Geometry check sheet. Reference: the model listing, model coordinates, mm. A direction names the side the tool comes from. Give positions to 0.01 mm unless a question says otherwise; leave off trailing zeros. Write each loop counter-clockwise with the first axis right and the second up, starting at its lowest first coordinate (ties: lowest second). Pieces come first, ordered by that corner, then holes. Notation, with made-up numbers: (-38, 32.5) -> (-19, 32.5) arc R15 ccw to (-19, 55.5) -> close; hole circle Ø6 at (-32.5, 78). An arc over 180 degrees is marked (long way). Use a Markdown table: item, result. Add a question column.
from build123d import *

# Parameters (mm, degrees)
SKETCH1_W           = 94
SKETCH1_H           = 130
BOSS_EXTRUDE1_DEPTH = 30
CUT_EXTRUDE2_DEPTH  = 23
SKETCH7_W           = 72
SKETCH7_H           = 24
CUT_EXTRUDE3_DEPTH  = 164.205392068
SKETCH8_W           = 6
SKETCH8_H           = 18
CUT_EXTRUDE4_DEPTH  = 4
SKETCH9_W           = 43
SKETCH9_H           = 8
CUT_EXTRUDE5_DEPTH  = 2.5
SKETCH10_W          = 70
SKETCH10_H          = 78
CUT_EXTRUDE6_DEPTH  = 2
SKETCH11_W          = 23
SKETCH11_H          = 3.5
CUT_EXTRUDE7_DEPTH  = 163.849623887
FILLET1_R           = 2
SKETCH12_R          = 5
CUT_EXTRUDE8_DEPTH  = 10


with BuildPart() as part:
    # Sketch1 → Boss-Extrude1 (new body)
    with BuildSketch(Plane(origin=(0, 0, 0), x_dir=(1, 0, 0), z_dir=(0, 1, 0))):
        with Locations((47, 65)):
            Rectangle(SKETCH1_W, SKETCH1_H)
    extrude(amount=BOSS_EXTRUDE1_DEPTH)

    # Sketch6 → Cut-Extrude2 (cut)
    with BuildSketch(Plane.XZ):
        Polygon((84, -125), (84, -120), (89, -120), (89, -10), (84, -10), (84, -5), (10, -5), (10, -10), (5, -10), (5, -120), (10, -120), (10, -125), align=None)
    extrude(amount=-CUT_EXTRUDE2_DEPTH, mode=Mode.SUBTRACT)

    # Sketch7 → Cut-Extrude3 (cut, through all)
    with BuildSketch(Plane(origin=(0, 30, 0), x_dir=(1, 0, 0), z_dir=(0, 1, 0))):
        with Locations((47, 100)):
            Rectangle(SKETCH7_W, SKETCH7_H)
    extrude(amount=-CUT_EXTRUDE3_DEPTH, mode=Mode.SUBTRACT)

    # Sketch8 → Cut-Extrude4 (cut)
    with BuildSketch(Plane.XZ.offset(-23)):
        with Locations((86, -100)):
            Rectangle(SKETCH8_W, SKETCH8_H)
    extrude(amount=-CUT_EXTRUDE4_DEPTH, mode=Mode.SUBTRACT)

    # Sketch9 → Cut-Extrude5 (cut)
    with BuildSketch(Plane.XZ.offset(-23)):
        with Locations((33.5, -116)):
            Rectangle(SKETCH9_W, SKETCH9_H)
    extrude(amount=-CUT_EXTRUDE5_DEPTH, mode=Mode.SUBTRACT)

    # Sketch10 → Cut-Extrude6 (cut)
    with BuildSketch(Plane(origin=(0, 30, 0), x_dir=(1, 0, 0), z_dir=(0, 1, 0))):
        with Locations((42, 44)):
            Rectangle(SKETCH10_W, SKETCH10_H)
    extrude(amount=-CUT_EXTRUDE6_DEPTH, mode=Mode.SUBTRACT)

    # Sketch11 → Cut-Extrude7 (cut, through all)
    with BuildSketch(Plane(origin=(0, 28, 0), x_dir=(1, 0, 0), z_dir=(0, 1, 0))):
        with Locations((42, 9.25)):
            Rectangle(SKETCH11_W, SKETCH11_H)
    extrude(amount=-CUT_EXTRUDE7_DEPTH, mode=Mode.SUBTRACT)

    # Fillet1
    fillet1_edges = [part.edges().sort_by_distance(p)[0] for p in [
        (94, 30, -65),
        (47, 30, -130),
        (0, 30, -65),
        (47, 30, 0),
        (0, 15, -130),
        (94, 15, -130),
        (94, 15, 0),
        (0, 15, 0),
    ]]
    fillet(fillet1_edges, radius=FILLET1_R)

    # Sketch12 → Cut-Extrude8 (cut)
    with BuildSketch(Plane.XY):
        with Locations((17.400096769, 12)):
            Circle(SKETCH12_R)
    extrude(amount=-CUT_EXTRUDE8_DEPTH, mode=Mode.SUBTRACT)


solid = part.part
1) Draft check along Z on faces 1 (the face through (30.5, 26, -9)), 2 (the face through (89, 13, -66)), 3 (the face through (46, 14, 0)), 4 (the face through (2, 0, -65)). Enter one of: +Z half, -Z half, draft (parallel to the pull), parting line (faces both ways), or undercut.
2) Sectioned sample at D-D, the plane z = -70. Enter the section's corners in (x, y), and give its area (3 significant figures).
3) Tool access check on faces 5 (the face through (33, 24, -120)), 6 (the face through (0, 14, -64)), 7 (the face through (42, 28, -45)), 8 (the face through (42, 26, -7.5)), 9 (the face through (47, 30, -84)). Record the directions out of +Z, -Z, +X, -X, +Y, -Y that give a thin tool (end or side, any length) a straight path to the whole face; none if there is none.
4) Sectioned sample at A-A, the plane x = 73. Enter the section's corners in (y, z).
5) Sectioned sample at B-B, the plane x = 32. Enter the section's corners in (y, z), and give its area (3 significant figures).
6) Material ranges on probe 1 along Z at (x, y) = (27, 16); probe 2 along X at (y, z) = (1.75, -34.5); probe 3 along X at (y, z) = (19.75, -7.5), recorded low to high. Write a range as [from, to].
7) Gauge pin test, flat ends, axial feed: P1, Ø0.6, axis at y = 29, z = -54.5, coming from the -X side; P2, Ø0.8, axis at x = 34.5, y = 24, coming from the +Z side. Record the tip position at first contact, or that the pin passes through.
8) Sectioned sample at C-C, the plane y = 3. Enter the section's corners in (x, z).
Check values:
| question | item | result |
|---|---|---|
| 1 | face 1 | undercut |
| 1 | face 2 | undercut |
| 1 | face 3 | +Z half |
| 1 | face 4 | draft |
| 2 | outline | (0, 0) -> (5, 0) -> (5, 23) -> (89, 23) -> (89, 0) -> (94, 0) -> (94, 28) arc R2 ccw to (92, 30) -> (77, 30) -> (77, 28) -> (7, 28) -> (7, 30) -> (2, 30) arc R2 ccw to (0, 28) -> close |
| 2 | area | 746 mm² |
| 3 | face 5 | -Y |
| 3 | face 6 | +Z, -Z, -X, +Y, -Y |
| 3 | face 7 | +Y |
| 3 | face 8 | +Y, -Y |
| 3 | face 9 | +Z, -Z, +X, -X, +Y |
| 4 | outline | (0, -130) -> (28, -130) arc R2 ccw to (30, -128) -> (30, -112) -> (23, -112) -> (23, -125) -> (0, -125) -> close; (0, -5) -> (23, -5) -> (23, -88) -> (30, -88) -> (30, -83) -> (28, -83) -> (28, -5) -> (30, -5) -> (30, -2) arc R2 ccw to (28, 0) -> (0, 0) -> close |
| 5 | outline | (0, -130) -> (28, -130) arc R2 ccw to (30, -128) -> (30, -112) -> (25.5, -112) -> (25.5, -120) -> (23, -120) -> (23, -125) -> (0, -125) -> close; (0, -5) -> (23, -5) -> (23, -7.5) -> (28, -7.5) -> (28, -5) -> (30, -5) -> (30, -2) arc R2 ccw to (28, 0) -> (0, 0) -> close; (23, -88) -> (30, -88) -> (30, -83) -> (28, -83) -> (28, -11) -> (23, -11) -> close |
| 5 | area | 777 mm² |
| 6 | probe 1 | [-130, -125], [-5, 0] |
| 6 | probe 2 | [0, 5], [89, 94] |
| 6 | probe 3 | [0, 10], [84, 94] |
| 7 | P1 | x = 0.13 |
| 7 | P2 | z = 0 |
| 8 | outline | (0, -128) arc R2 ccw to (2, -130) -> (92, -130) arc R2 ccw to (94, -128) -> (94, -2) arc R2 ccw to (92, 0) -> (2, 0) arc R2 ccw to (0, -2) -> close; hole (5, -120) -> (10, -120) -> (10, -125) -> (84, -125) -> (84, -120) -> (89, -120) -> (89, -10) -> (84, -10) -> (84, -5) -> (10, -5) -> (10, -10) -> (5, -10) -> close |
